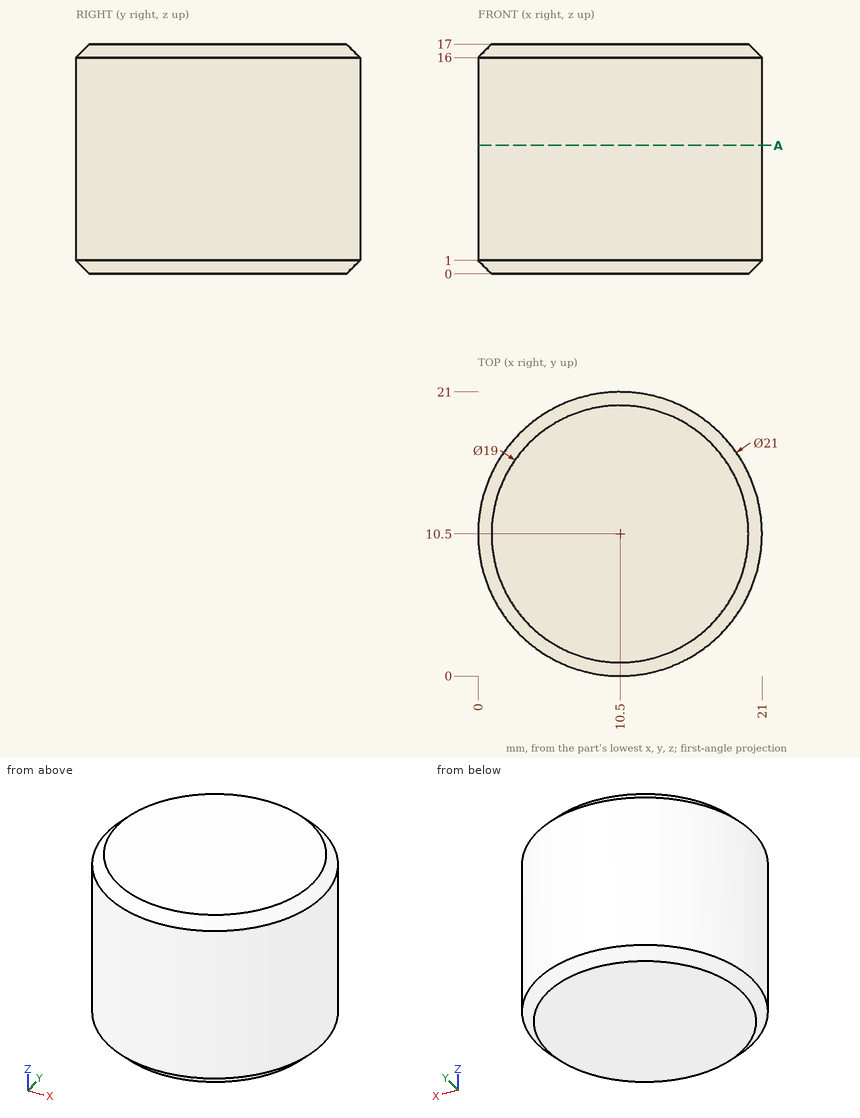
Input: dimensioned drawing with shaded views. Units: mm. Origin: part minimum x, y, z. Coordinates: 2 decimals unless noted, no trailing zeros. Order: outer loops, then holes, each group sorted by start corner. A loop starts at its lowest first (then second) coordinate and runs counter-clockwise, first axis right, second up.
(1) First-contact query: pin 1 (10 mm diameter, centred on y = 2.5, z = 15, fed in from +X); pin 2 (3 mm diameter, centred on y = 14.5, z = 5.5, fed in from -X); pin 3 (4 mm diameter, centred on x = 7.5, z = 9.5, fed in from +Y). Flat tips, straight axial feed; report the tip coordinate or a pass-through.
(2) Section query A-A (z = 9.5). Return the cut outline in (x, y), plus the area to 3 significant figures.
(3) Material intervals for probe 1 along Y at (x, z) = (10.75, 4.75); probe 2 along X at (y, z) = (19.75, 8); probe 3 along Y at (x, z) = (13.5, 9), sorted ascending.
Solution:
1. pin 1: stops at x = 20.56
1. pin 2: stops at x = 0.3
1. pin 3: stops at y = 20.95
2. outline: circle Ø21 at (10.5, 10.5)
2. area: 346 mm2
3. probe 1: y = 0 to 21
3. probe 2: x = 5.53 to 15.47
3. probe 3: y = 0.44 to 20.56
